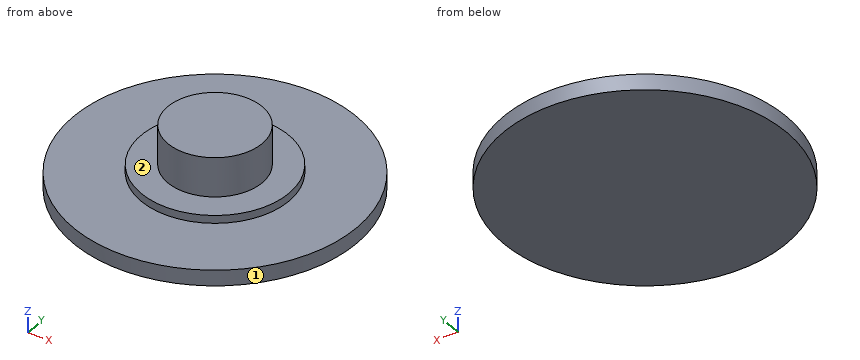
```python
from build123d import *

# Parameters (mm, degrees)
F0_R     = 3
F1_DEPTH = 4
F0_R_2   = 9
F0_R_3   = 4.7
F2_DEPTH = 1
F3_DEPTH = 1.5


with BuildPart() as f1:
    # F0 (on Top) → F1 (new body)
    with BuildSketch(Plane.XY):
        Circle(F0_R)
    extrude(amount=F1_DEPTH)



with BuildPart() as f2:
    # F0 (on Top) → F2 (new body)
    with BuildSketch(Plane.XY):
        Circle(F0_R_2)
        Circle(F0_R_3, mode=Mode.SUBTRACT)
    extrude(amount=F2_DEPTH)


with BuildPart() as f1_1:
    add(f1.part)

    add(f2.part)  # F3 merges F2
    # F0 (on Top) → F3 (join)
    with BuildSketch(Plane.XY):
        Circle(F0_R_3)
        Circle(F0_R, mode=Mode.SUBTRACT)
    extrude(amount=F3_DEPTH)


solid = f1_1.part
```
Geometry check sheet. Reference: the model listing, model coordinates, mm. Face numbers are marked on the shaded views. A direction names the side the tool comes from. Coordinates: 2 decimals unless noted, no trailing zeros. Order: outer loops, then holes, each group sorted by start corner. A loop starts at its lowest first (then second) coordinate and runs counter-clockwise, first axis right, second up.
Item 1: Tool access check on the marked faces 1 and 2. Record the directions out of +Z, -Z, +X, -X, +Y, -Y that give a thin tool (end or side, any length) a straight path to the whole face; none if there is none.
Item 2: Scan lines: line 1 along Z through (x, y) = (5.25, 4); line 2 along Z through (x, y) = (-3.25, 0.5); line 3 along Y through (x, z) = (6.75, 0.4). Record each from-to range of solid material in increasing order.
Item 3: Section check C-C (x = 7). Enter the section's corners in (y, z), plus the area to 3 significant figures.
Item 4: Section check A-A (x = 0). Enter the section's corners in (y, z), plus the area to 3 significant figures.
Item 5: Section check D-D (x = -6.75). Enter the section's corners in (y, z), plus the area to 3 significant figures.
Item 6: Depth check by flat-ended pin: pin 1 (1 mm diameter, centred on x = 7, y = 2.5, fed in from +Z); pin 2 (4 mm diameter, centred on x = 2.5, y = 5.5, fed in from -Z); pin 3 (1.5 mm diameter, centred on x = -1, z = 0.5, fed in from +Y). Enter the tip coordinate at first touch or a pass-through.
Check sheet entries:
1. face 1: +Z, -Z
1. face 2: +Z
2. line 1: z = 0 to 1
2. line 2: z = 0 to 1.5
2. line 3: y = -5.95 to 5.95
3. outline: (-5.66, 0) - (5.66, 0) - (5.66, 1) - (-5.66, 1) - close
3. area: 11.3 mm2
4. outline: (-9, 0) - (9, 0) - (9, 1) - (4.7, 1) - (4.7, 1.5) - (3, 1.5) - (3, 4) - (-3, 4) - (-3, 1.5) - (-4.7, 1.5) - (-4.7, 1) - (-9, 1) - close
4. area: 37.7 mm2
5. outline: (-5.95, 0) - (5.95, 0) - (5.95, 1) - (-5.95, 1) - close
5. area: 11.9 mm2
6. pin 1: stops at z = 1
6. pin 2: stops at z = 0
6. pin 3: stops at y = 9
